from build123d import *

# Parameters (mm, degrees)
SKETCH_R     = 12
PAD_DEPTH    = 3
SKETCH001_R  = 10
POCKET_DEPTH = 2.5
FILLET_R     = 0.4


with BuildPart() as part:
    # Sketch → Pad (new body)
    with BuildSketch(Plane.XY):
        Circle(SKETCH_R)
    extrude(amount=PAD_DEPTH)

    # Sketch001 → Pocket (cut)
    with BuildSketch(Plane.XY):
        with Locations((0, -2.467762)):
            Circle(SKETCH001_R)
    extrude(amount=POCKET_DEPTH, mode=Mode.SUBTRACT)

    # Fillet
    fillet_edges = [part.edges().sort_by_distance(p)[0] for p in [
        (-12, 0, 3),
        (-4.240751, 6.588508, 0),
        (-5.794891, 10.508056, 0),
        (9.05627, -6.708513, 0),
        (-6.403207, -10.14884, 1.25),
        (6.403207, -10.14884, 1.25),
    ]]
    fillet(fillet_edges, radius=FILLET_R)


solid = part.part
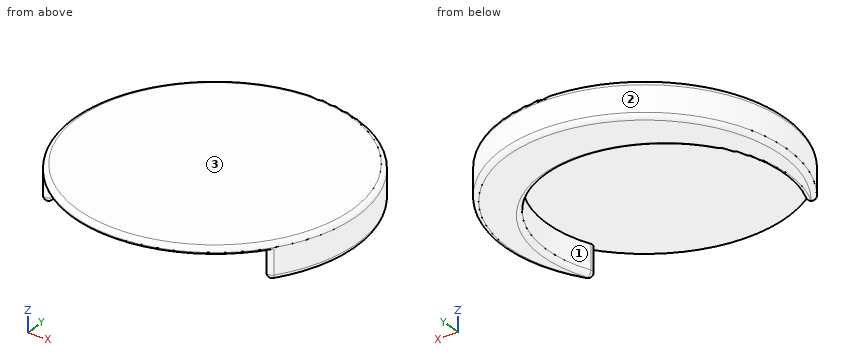
Geometry check sheet. Reference: the model listing, model coordinates, mm. Face numbers are marked on the shaded views. Round coordinates to 2 decimals unless told otherwise and drop trailing zeros. Order: outer loops, then holes, each group sorted by start corner. A loop starts at its lowest first (then second) coordinate and runs counter-clockwise, first axis right, second up. Notation, with made-up numbers: M -14.75,88 L -4.75,88 A16 cw -4.75,92 Z; hole C 31.25,31 d3. An arc over 180 degrees is marked long. Write each question's results on one line, items separated by ' | '. Start each with the question number.
1. Go/stop test with flat-tipped pins: P1, Ø1.5, axis at x = 2, z = 2.5, coming from the -Y side; P2, Ø1, axis at x = -4, z = 2.5, coming from the -Y side. Record where each tip stops, or that it passes through.
2. Draft check along X on the marked faces 1, 2 and 3. Enter one of: pulls with the +X half, pulls with the -X half, needs draft (parallel to the pull), parting line crosses it, or undercut.
3. Material ranges on L1, parallel to Z at x = -4.5, y = 4.5; L2, parallel to X at y = -3.75, z = 0.8; L3, parallel to X at y = 0, z = 0.9, recorded low to high. Write a range as from..to.
4. Cross-section at A-A on x = 0. Record the boundary of the cut face in (y, z).
Resolved:
1) P1: y = -11.93 | P2: y = -11.48
2) face 1: undercut | face 2: parting line crosses it | face 3: needs draft
3) L1: 2.5..3 | L2: -11.4..-9.92, 9.92..11.4 | L3: -12..-9.69, 9.69..12
4) outline: M -12,2.5 L 7.53,2.5 L 7.53,0.4 A0.4 ccw 7.93,0 L 11.6,0 A0.4 ccw 12,0.4 L 12,2.6 A0.4 ccw 11.6,3 L -11.6,3 A0.4 ccw -12,2.6 Z
